```python
from build123d import *

# Parameters (mm, degrees)
BOSS_EXTRUDE1_DEPTH = 2.8
SKETCH2_R           = 2.1
CUT_EXTRUDE1_DEPTH  = 103.897230283
FILLET1_R           = 6
CHAMFER2_SIZE       = 4.28444402
CHAMFER2_SIZE_2     = 3
FILLET2_R           = 3


with BuildPart() as part:
    # Sketch1 → Boss-Extrude1 (new body)
    with BuildSketch(Plane(origin=(0, 0, 0), x_dir=(1, 0, 0), z_dir=(0, 1, 0))):
        Polygon((0, 4), (40, 4), (70, 0), (92, 0), (88, -46), (0, -46), (-8, -46), (-8, -28), (0, -20), align=None)
    extrude(amount=BOSS_EXTRUDE1_DEPTH)

    # Sketch2 → Cut-Extrude1 (cut, through all)
    with BuildSketch(Plane(origin=(0, 2.8, 0), x_dir=(1, 0, 0), z_dir=(0, 1, 0))):
        with Locations(Location((7, -6, 0), (0, 0, 270))):
            Circle(SKETCH2_R)
        with Locations(Location((7, -29, 0), (0, 0, 270))):
            Circle(SKETCH2_R)
        with Locations(Location((73, -6, 0), (0, 0, 270))):
            Circle(SKETCH2_R)
        with Locations(Location((73, -29, 0), (0, 0, 270))):
            Circle(SKETCH2_R)
    extrude(amount=-CUT_EXTRUDE1_DEPTH, mode=Mode.SUBTRACT)

    # Fillet1
    fillet1_edges = [part.edges().sort_by_distance(p)[0] for p in [
        (-8, 1.4, 28),
        (0, 1.4, 20),
    ]]
    fillet(fillet1_edges, radius=FILLET1_R)

    # Chamfer2
    # the kernel refuses this chamfer: 4.28444402, 3 mm, written as the material it takes off along each edge
    with BuildSketch(Plane(origin=(99.06480046, 2.8, 46), x_dir=(0, 0.02220967419845692, -0.99975333476413), z_dir=(-1, 0, 0))) as chamfer2_piece_1:
        Polygon((CHAMFER2_SIZE * 0.999753334817, CHAMFER2_SIZE * 0.0222096741996), (-CHAMFER2_SIZE_2 * 0.0222096741985, CHAMFER2_SIZE_2 * 0.999753334764), (0, 0), align=None)
    extrude(amount=118.12960092, mode=Mode.SUBTRACT)

    # Fillet2
    fillet2_edges = [part.edges().sort_by_distance(p)[0] for p in [
        (0, 1.4, -4),
        (92, 1.4, 0),
    ]]
    fillet(fillet2_edges, radius=FILLET2_R)


solid = part.part
```
The listing builds one solid part. Answer for the finished solid, in the listing's coordinates (mm). A direction names the side the tool comes from. Round coordinates to 2 decimals unless told otherwise and drop trailing zeros. Loops run counter-clockwise (first coordinate to the right, second up) from the corner with the lowest first, then second, coordinate; pieces in that order, holes last. Notation, with made-up numbers: (-31, 82.5) - (20, 82.5) arc R14 cw to (20, 100.5) - close; hole circle Ø10 at (-11, 16). An arc over 180 degrees is marked (long way). Return JSON: item names as keys, results as strings. Group by question number.
1. Which of the six approach directions +Z, -Z, +X, -X, +Y, -Y give full straight-line access (tool end or side, diameter ignored) to faces 1 (the flat face through (79, 1, 0)), 2 (the cylindrical face through (9.082, 1.42, 5.727)), 3 (the flat face through (0, 1, 8))?
2. The part is cut by section C-C on y = 1.55. Determine the outline of the cut face in (x, z).
3. The part is cut by section A-A on z = 29. Determine the outline of the cut face in (x, y), then the cut area to 3 significant figures.
4. The mould has two halves that part along X. Classify faces 4 (the flat face through (89.897, 1.38, 24.19)), 5 (the cylindrical face through (8.419, 1.42, 27.452)), 6 (the cylindrical face through (71.722, 1.42, 27.334)), 7 (the flat face through (-8, 1, 37)): pulls with the +X half, pulls with the -X half, needs draft (parallel to the pull), parting line crosses it, or undercut.
5. This flat-tipped pin is pushed along its axis until it touches: P1, Ø5, axis at x = 73, z = 29, coming from the -Y side. Where does it stop, or does it pass through?
6. The part is cut by section B-B on x = 73. Determine the outline of the cut face in (y, z), then the cut area to 3 significant figures.
7. Consider probe 1 along X at (y, z) = (2.1, 27.5); probe 2 along X at (y, z) = (1.55, 6); probe 3 along Z at (x, y) = (48, 1.3). Determine where each line is inside the solid, lowest interval first.
8. The part is cut by section D-D on z = 20.5. Determine the outline of the cut face in (x, y), then the cut area to 3 significant figures.
Resolved:
{
 "1": {"face 1": "-Z, +X, +Y, -Y", "face 2": "+Y, -Y", "face 3": "-Z, -X, +Y, -Y"},
 "2": {"outline": "(-8, 30.49) arc R6 ccw to (-6.24, 26.24) - (-1.76, 21.76) arc R6 cw to (0, 17.51) - (0, -1) arc R3 ccw to (3, -4) - (40, -4) - (70, 0) - (88.73, 0) arc R3 ccw to (91.72, 3.26) - (88.22, 43.5) - (-8, 43.5) - close; hole circle Ø4.2 at (7, 6); hole circle Ø4.2 at (7, 29); hole circle Ø4.2 at (73, 6); hole circle Ø4.2 at (73, 29)"},
 "3": {"outline": "(-7.81, 0) - (4.9, 0) - (4.9, 2.8) - (-7.81, 2.8) - close; (9.1, 0) - (70.9, 0) - (70.9, 2.8) - (9.1, 2.8) - close; (75.1, 0) - (89.48, 0) - (89.48, 2.8) - (75.1, 2.8) - close", "area": "249 mm²"},
 "4": {"face 4": "pulls with the +X half", "face 5": "undercut", "face 6": "undercut", "face 7": "pulls with the -X half"},
 "5": {"P1": "stops at y = 0"},
 "6": {"outline": "(0, 0) - (2.8, 0) - (2.8, 3.9) - (0, 3.9) - close; (0, 8.1) - (2.8, 8.1) - (2.8, 26.9) - (0, 26.9) - close; (0, 31.1) - (2.8, 31.1) - (2.8, 41.72) - (0, 45.71) - close", "area": "98.9 mm²"},
 "7": {"probe 1": "x = -7.2 to 5.53, 8.47 to 71.53, 74.47 to 89.61", "probe 2": "x = 0 to 4.9, 9.1 to 70.9, 75.1 to 91.48", "probe 3": "z = -2.93 to 43.86"},
 "8": {"outline": "(-0.8, 0) - (90.22, 0) - (90.22, 2.8) - (-0.8, 2.8) - close", "area": "255 mm²"}
}
